Verification items for the finished model (mm, model axes). A direction names the side the tool comes from. Coordinates: 2 decimals unless noted, no trailing zeros. Write each loop counter-clockwise with the first axis right and the second up, starting at its lowest first coordinate (ties: lowest second). Pieces come first, ordered by that corner, then holes. Notation, with made-up numbers: M 75,65 L 121,65 A22 ccw 121,81 Z; hole C 68.25,-22 d3. An arc over 180 degrees is marked long. Answer in a Markdown table with one row per item.
from build123d import *

# Parameters (mm, degrees)
PAD_DEPTH = 30


with BuildPart() as part:
    # Sketch → Pad (new body)
    with BuildSketch(Plane.XY):
        with BuildLine():
            Line((54, 22.909644), (54, 49.60153))
            ThreePointArc((54, 49.60153), (52.594283, 52.995232), (49.200581, 54.400949))
            Line((49.200581, 54.400949), (4.409496, 54.400949))
            ThreePointArc((4.409496, 54.400949), (1.291512, 53.109437), (0, 49.991452))
            Line((0, 49.991452), (0, -56.197297))
            ThreePointArc((-1.5, -57.697297), (-0.43934, -57.257957), (0, -56.197297))
            Line((-1.5, -57.697297), (-31.710882, -57.697297))
            ThreePointArc((-33.210882, -56.197297), (-32.771543, -57.257957), (-31.710882, -57.697297))
            Line((-33.210882, -56.197297), (-33.210882, -35.774231))
            Line((-33.210934, -35.774231), (-33.210882, -35.774231))
            ThreePointArc((-33.210934, -35.774231), (-34.710834, -34.265328), (-36.210882, -35.774084))
            Line((-36.210882, -56.506556), (-36.210882, -35.774084))
            ThreePointArc((-36.210882, -56.506556), (-34.983443, -59.469857), (-32.020141, -60.697297))
            Line((-1.418408, -60.697297), (-32.020141, -60.697297))
            ThreePointArc((-1.418408, -60.697297), (1.705878, -59.403175), (3, -56.278889))
            Line((3, 49.900949), (3, -56.278889))
            ThreePointArc((4.5, 51.400949), (3.43934, 50.961609), (3, 49.900949))
            Line((49.5, 51.400949), (4.5, 51.400949))
            ThreePointArc((51, 49.900949), (50.56066, 50.961609), (49.5, 51.400949))
            Line((51, 22.909644), (51, 49.900949))
            ThreePointArc((51, 22.909644), (52.5, 21.409644), (54, 22.909644))
        make_face()
    extrude(amount=PAD_DEPTH)


solid = part.part
1) Sectioned sample at D-D (y = 12.5). Record the cut outline in (x, z).
Response values:
| item | result |
|---|---|
| outline | M 0,0 L 3,0 L 3,30 L 0,30 Z |
2) Sectioned sample at C-C (x = 14). Record the cut outline in (y, z).
Response values:
| item | result |
|---|---|
| outline | M 51.4,0 L 54.4,0 L 54.4,30 L 51.4,30 Z |
3) Tool access check on faces 5 (the face through (2, 1, 30)), 6 (the face through (0, -2, 15)), 7 (the face through (27, 51.401, 15)). Record the directions out of +Z, -Z, +X, -X, +Y, -Y that give a thin tool (end or side, any length) a straight path to the whole face; none if there is none.
Response values:
| item | result |
|---|---|
| face 5 | +Z, +X, -X, +Y, -Y |
| face 6 | +Z, -Z, +Y |
| face 7 | +Z, -Z, -Y |
4) Thickness scan on L1, parallel to X at y = 37.5, z = 10.5; L2, parallel to X at y = -38, z = 10.5; L3, parallel to X at y = -24, z = 26. Record the ranges inside material, lowest first. Write a range as [from, to].
Response values:
| item | result |
|---|---|
| L1 | x = [0, 3], [51, 54] |
| L2 | x = [-36.21, -33.21], [0, 3] |
| L3 | x = [0, 3] |
5) Sectioned sample at A-A (y = -44.5). Record the cut outline in (x, z), then the cut area to 3 significant figures.
Response values:
| item | result |
|---|---|
| outline | M -36.21,0 L -33.21,0 L -33.21,30 L -36.21,30 Z; M 0,0 L 3,0 L 3,30 L 0,30 Z |
| area | 180 mm² |
6) Depth check by flat-ended pin: pin 1 (10 mm diameter, centred on y = -50, z = 16.5, fed in from +X); pin 2 (3 mm diameter, centred on x = 8, z = 11, fed in from -Y); pin 3 (8 mm diameter, centred on y = 43, z = 20, fed in from -X). Enter the tip coordinate at first touch or a pass-through.
Response values:
| item | result |
|---|---|
| pin 1 | stops at x = 3 |
| pin 2 | stops at y = 51.4 |
| pin 3 | stops at x = 0 |
7) Release check for a two-part mould opening along X. For faces 1 (the face through (-36.211, -46, 15)), 2 (the face through (-33.211, -46, 15)), 3 (the face through (54, 36, 15)), 4 (the face through (3, -2, 15)) record: +X half, -X half, draft (parallel to the pull), parting line (faces both ways), or undercut.
Response values:
| item | result |
|---|---|
| face 1 | -X half |
| face 2 | undercut |
| face 3 | +X half |
| face 4 | undercut |
